The model under review builds one solid part; all positions refer to its coordinate system, in mm. Coordinates: 2 decimals unless noted, no trailing zeros. Write each loop counter-clockwise with the first axis right and the second up, starting at its lowest first coordinate (ties: lowest second). Pieces come first, ordered by that corner, then holes. Notation, with made-up numbers: (52, 57.5) - (97, 57.5) arc R17 cw to (97, 62.5) - close; hole circle Ø10 at (58, 41.5). An arc over 180 degrees is marked (long way). Put each result on its own line as item: value. Start each with the question number.
Item 1: To check wall thickness, follow L1, parallel to X at y = -0.55, z = -13.5; L2, parallel to Z at x = -1.5, y = 1.05; L3, parallel to Z at x = 4, y = -1.2. State the ranges of each line that lie inside material, in increasing order. Write a range as [from, to].
Item 2: Consider section C-C on z = 41.5. Give the boundary of the cut face in (x, y), then the cut area to 3 significant figures.
Item 3: Mouldability with a two-part tool opening along Z and no side actions: class faces 1 (the face through (-69.184, 0.028, 15.15)), 2 (the face through (1, 2, -1)), 3 (the face through (72.556, 0.028, -13)), 4 (the face through (-51.721, 0.028, -67.453)) as pulls with the +Z half, pulls with the -Z half, needs draft (parallel to the pull), parting line crosses it, or undercut.
Item 4: Consider section B-B on y = 0.25. Give the boundary of the cut face in (x, z) (3 decimals), then the cut area to 3 significant figures.
Item 5: For pin 1 (1.5 mm diameter, centred on y = 0, z = 53.5, fed in from +X); pin 2 (2.5 mm diameter, centred on x = -70.87, z = -14.075, fed in from -Y); pin 3 (2 mm diameter, centred on x = 5.5, y = -1, fed in from -Z), all flat-tipped, find the tip position at first contact; note any pin that passes through.
Item 6: Consider section A-A on x = 70.87. Give the boundary of the cut face in (y, z) (3 decimals), then the cut area to 3 significant figures.
Item 7: Consider section D-D on x = -40.5. Give the boundary of the cut face in (y, z).
```python
from build123d import *

# Parameters (mm, degrees)
SKETCH1_R           = 85
BOSS_EXTRUDE1_DEPTH = 2
SKETCH2_R           = 2
CUT_EXTRUDE1_DEPTH  = 121.274685616


with BuildPart() as part:
    # Sketch1 → Boss-Extrude1 (new, symmetric)
    with BuildSketch(Plane(origin=(0, 0, 0), x_dir=(1, 0, 0), z_dir=(0, 1, 0))):
        with Locations(Location((0, 0, 0), (0, 0, 270))):
            Circle(SKETCH1_R)
    extrude(amount=BOSS_EXTRUDE1_DEPTH, both=True)

    # Sketch2 → Cut-Extrude1 (cut, through all)
    with BuildSketch(Plane(origin=(0, 2, 0), x_dir=(1, 0, 0), z_dir=(0, 1, 0))):
        with Locations(Location((70.87, 14.075, 0), (0, 0, 270))):
            Circle(SKETCH2_R)
        with Locations(Location((70.87, -14.075, 0), (0, 0, 90))):
            Circle(SKETCH2_R)
        with Locations(Location((-70.87, -14.075, 0), (0, 0, 270))):
            Circle(SKETCH2_R)
        with Locations(Location((-70.87, 14.075, 0), (0, 0, 90))):
            Circle(SKETCH2_R)
    extrude(amount=-CUT_EXTRUDE1_DEPTH, mode=Mode.SUBTRACT)


solid = part.part
```
Report:
1. L1: [-83.92, -72.79], [-68.95, 68.95], [72.79, 83.92]
1. L2: [-84.99, 84.99]
1. L3: [-84.91, 84.91]
2. outline: (-74.18, -2) - (74.18, -2) - (74.18, 2) - (-74.18, 2) - close
2. area: 593 mm²
3. face 1: undercut
3. face 2: needs draft
3. face 3: undercut
3. face 4: parting line crosses it
4. outline: circle Ø170 at (0, 0); hole circle Ø4 at (-70.87, -14.075); hole circle Ø4 at (-70.87, 14.075); hole circle Ø4 at (70.87, -14.075); hole circle Ø4 at (70.87, 14.075)
4. area: 22,600 mm²
5. pin 1: x = 66.65
5. pin 2: through
5. pin 3: z = -84.88
6. outline: (-2, -46.93) - (2, -46.93) - (2, -16.075) - (-2, -16.075) - close; (-2, -12.075) - (2, -12.075) - (2, 12.075) - (-2, 12.075) - close; (-2, 16.075) - (2, 16.075) - (2, 46.93) - (-2, 46.93) - close
6. area: 343 mm²
7. outline: (-2, -74.73) - (2, -74.73) - (2, 74.73) - (-2, 74.73) - close
